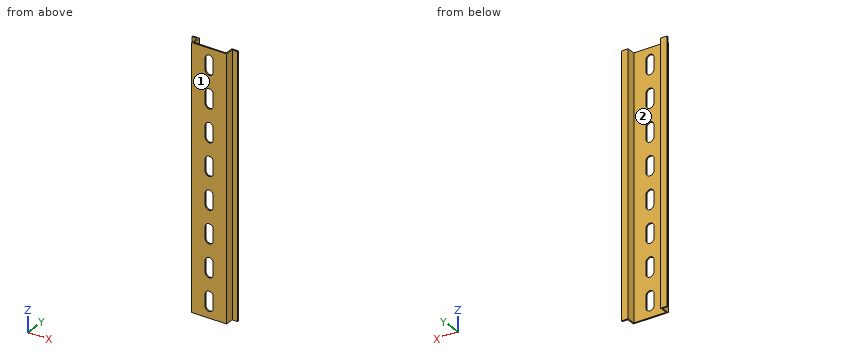
```python
from build123d import *

# Parameters (mm, degrees)
BOSS_EXTRUDE1_DEPTH  = 200
CUT_EXTRUDE1_DEPTH   = 201.904206029
LPATTERN1_COUNT      = 8
LPATTERN1_PITCH      = 25
MIRROR2_COPY_1_DEPTH = 201.904206029
MIRROR2_COPY_2_DEPTH = 201.904206029
MIRROR2_COPY_3_DEPTH = 201.904206029
MIRROR2_COPY_4_DEPTH = 201.904206029
MIRROR2_COPY_5_DEPTH = 201.904206029
MIRROR2_COPY_6_DEPTH = 201.904206029
MIRROR2_COPY_7_DEPTH = 201.904206029


with BuildPart() as part:
    # Sketch1 → Boss-Extrude1 (new body)
    with BuildSketch(Plane.XY):
        Polygon((0, 0), (13.5, 0), (13.5, 6.5), (17.5, 6.5), (17.5, 7.5), (12.5, 7.5), (12.5, 1), (0, 1), align=None)
    boss_extrude1 = extrude(amount=BOSS_EXTRUDE1_DEPTH)

    # Sketch2 → Cut-Extrude1 (cut, through all)
    with BuildSketch(Plane(origin=(0, 0, 0), x_dir=(1, 0, 0), z_dir=(0, 1, 0))):
        with BuildLine():
            Line((3.1, -8.1), (3.1, -16.9))
            ThreePointArc((3.1, -16.9), (0, -20), (-3.1, -16.9))
            Line((-3.1, -16.9), (-3.1, -8.1))
            ThreePointArc((-3.1, -8.1), (0, -5), (3.1, -8.1))
        make_face()
    cut_extrude1 = extrude(amount=CUT_EXTRUDE1_DEPTH, mode=Mode.SUBTRACT)

    # LPattern1: Cut-Extrude1 ×8
    with Locations(*[(0, 0, i * LPATTERN1_PITCH) for i in range(1, LPATTERN1_COUNT)]):
        add(cut_extrude1, mode=Mode.SUBTRACT)

    # Mirror2: Boss-Extrude1, Cut-Extrude1 across plane
    add(boss_extrude1.mirror(Plane(origin=(0, 0, 0), x_dir=(0, 0, 1), z_dir=(1, 0, 0))))
    add(cut_extrude1.mirror(Plane(origin=(0, 0, 0), x_dir=(0, 0, 1), z_dir=(1, 0, 0))), mode=Mode.SUBTRACT)

    # Mirror2 copy 1 sketch → Mirror2 copy 1 (cut, through all)
    with BuildSketch(Plane(origin=(0, 0, 25), x_dir=(-1, 0, 0), z_dir=(0, 1, 0))):
        with BuildLine():
            Line((3.1, 8.1), (3.1, 16.9))
            ThreePointArc((3.1, 16.9), (0, 20), (-3.1, 16.9))
            Line((-3.1, 16.9), (-3.1, 8.1))
            ThreePointArc((-3.1, 8.1), (0, 5), (3.1, 8.1))
        make_face()
    extrude(amount=MIRROR2_COPY_1_DEPTH, mode=Mode.SUBTRACT)

    # Mirror2 copy 2 sketch → Mirror2 copy 2 (cut, through all)
    with BuildSketch(Plane(origin=(0, 0, 50), x_dir=(-1, 0, 0), z_dir=(0, 1, 0))):
        with BuildLine():
            Line((3.1, 8.1), (3.1, 16.9))
            ThreePointArc((3.1, 16.9), (0, 20), (-3.1, 16.9))
            Line((-3.1, 16.9), (-3.1, 8.1))
            ThreePointArc((-3.1, 8.1), (0, 5), (3.1, 8.1))
        make_face()
    extrude(amount=MIRROR2_COPY_2_DEPTH, mode=Mode.SUBTRACT)

    # Mirror2 copy 3 sketch → Mirror2 copy 3 (cut, through all)
    with BuildSketch(Plane(origin=(0, 0, 75), x_dir=(-1, 0, 0), z_dir=(0, 1, 0))):
        with BuildLine():
            Line((3.1, 8.1), (3.1, 16.9))
            ThreePointArc((3.1, 16.9), (0, 20), (-3.1, 16.9))
            Line((-3.1, 16.9), (-3.1, 8.1))
            ThreePointArc((-3.1, 8.1), (0, 5), (3.1, 8.1))
        make_face()
    extrude(amount=MIRROR2_COPY_3_DEPTH, mode=Mode.SUBTRACT)

    # Mirror2 copy 4 sketch → Mirror2 copy 4 (cut, through all)
    with BuildSketch(Plane(origin=(0, 0, 100), x_dir=(-1, 0, 0), z_dir=(0, 1, 0))):
        with BuildLine():
            Line((3.1, 8.1), (3.1, 16.9))
            ThreePointArc((3.1, 16.9), (0, 20), (-3.1, 16.9))
            Line((-3.1, 16.9), (-3.1, 8.1))
            ThreePointArc((-3.1, 8.1), (0, 5), (3.1, 8.1))
        make_face()
    extrude(amount=MIRROR2_COPY_4_DEPTH, mode=Mode.SUBTRACT)

    # Mirror2 copy 5 sketch → Mirror2 copy 5 (cut, through all)
    with BuildSketch(Plane(origin=(0, 0, 125), x_dir=(-1, 0, 0), z_dir=(0, 1, 0))):
        with BuildLine():
            Line((3.1, 8.1), (3.1, 16.9))
            ThreePointArc((3.1, 16.9), (0, 20), (-3.1, 16.9))
            Line((-3.1, 16.9), (-3.1, 8.1))
            ThreePointArc((-3.1, 8.1), (0, 5), (3.1, 8.1))
        make_face()
    extrude(amount=MIRROR2_COPY_5_DEPTH, mode=Mode.SUBTRACT)

    # Mirror2 copy 6 sketch → Mirror2 copy 6 (cut, through all)
    with BuildSketch(Plane(origin=(0, 0, 150), x_dir=(-1, 0, 0), z_dir=(0, 1, 0))):
        with BuildLine():
            Line((3.1, 8.1), (3.1, 16.9))
            ThreePointArc((3.1, 16.9), (0, 20), (-3.1, 16.9))
            Line((-3.1, 16.9), (-3.1, 8.1))
            ThreePointArc((-3.1, 8.1), (0, 5), (3.1, 8.1))
        make_face()
    extrude(amount=MIRROR2_COPY_6_DEPTH, mode=Mode.SUBTRACT)

    # Mirror2 copy 7 sketch → Mirror2 copy 7 (cut, through all)
    with BuildSketch(Plane(origin=(0, 0, 175), x_dir=(-1, 0, 0), z_dir=(0, 1, 0))):
        with BuildLine():
            Line((3.1, 8.1), (3.1, 16.9))
            ThreePointArc((3.1, 16.9), (0, 20), (-3.1, 16.9))
            Line((-3.1, 16.9), (-3.1, 8.1))
            ThreePointArc((-3.1, 8.1), (0, 5), (3.1, 8.1))
        make_face()
    extrude(amount=MIRROR2_COPY_7_DEPTH, mode=Mode.SUBTRACT)


solid = part.part
```
CAD build for the part. Positions are in the model's coordinates, mm. Face numbers are marked on the shaded views. A direction names the side the tool comes from. Coordinates: 2 decimals unless noted, no trailing zeros. Order: outer loops, then holes, each group sorted by start corner. A loop starts at its lowest first (then second) coordinate and runs counter-clockwise, first axis right, second up. Notation, with made-up numbers: (-26, 82.5) - (22, 82.5) arc R22 cw to (22, 97.5) - close; hole circle Ø3 at (18, 48.5). An arc over 180 degrees is marked (long way). Answer in a Markdown table with one row per item.
1. Slice it at D-D, the plane x = 8.5. List the corners of the cut face in (y, z).
Answer:
| item | result |
|---|---|
| outline | (0, 0) - (1, 0) - (1, 200) - (0, 200) - close |
2. Drill centre lines: L1, parallel to X at y = 5.75, z = 156; L2, parallel to X at y = 0.5, z = 64.5; L3, parallel to Y at x = 9, z = 149.5. Where is each one in solid material? Low to high. Write a range as from..to.
Answer:
| item | result |
|---|---|
| L1 | -13.5..-12.5, 12.5..13.5 |
| L2 | -13.5..-3.1, 3.1..13.5 |
| L3 | 0..1 |
3. Slice it at A-A, the plane y = 3. List the corners of the cut face in (x, z), then the cut area to 3 significant figures.
Answer:
| item | result |
|---|---|
| outline | (-13.5, 0) - (-12.5, 0) - (-12.5, 200) - (-13.5, 200) - close; (12.5, 0) - (13.5, 0) - (13.5, 200) - (12.5, 200) - close |
| area | 400 mm² |
4. Flat gauge pins, fed straight in: P1, Ø1.1, axis at y = 0.5, z = 88, coming from the +X side; P2, Ø6, axis at x = 4, z = 64, coming from the +Y side; P3, Ø0.5, axis at y = 0.5, z = 189, coming from the -X side; P4, Ø1.5, axis at x = 0, z = 57, coming from the +Y side. Where does each tip first touch, or does it go through?
Answer:
| item | result |
|---|---|
| P1 | x = 13.5 |
| P2 | y = 1 |
| P3 | x = -13.5 |
| P4 | through |
5. Slice it at B-B, the plane z = 24. List the corners of the cut face in (x, y).
Answer:
| item | result |
|---|---|
| outline | (-17.5, 6.5) - (-13.5, 6.5) - (-13.5, 0) - (13.5, 0) - (13.5, 6.5) - (17.5, 6.5) - (17.5, 7.5) - (12.5, 7.5) - (12.5, 1) - (-12.5, 1) - (-12.5, 7.5) - (-17.5, 7.5) - close |
6. 3-axis set-ups, long thin cutter, end or side, ignore diameter. For the marked faces 1 and 2: which of +Z, -Z, +X, -X, +Y, -Y reach the whole face in a straight line?
Answer:
| item | result |
|---|---|
| face 1 | +Z, -Z, +X, -X, -Y |
| face 2 | +Z, -Z, +Y |
7. Slice it at C-C, the plane x = 0. Give the number of separate pieces and of enclosed holes in the cut face, then the cut area to 3 significant figures.
Answer:
| item | result |
|---|---|
| separate pieces | 9 |
| enclosed holes | 0 |
| area | 80.0 mm² |
